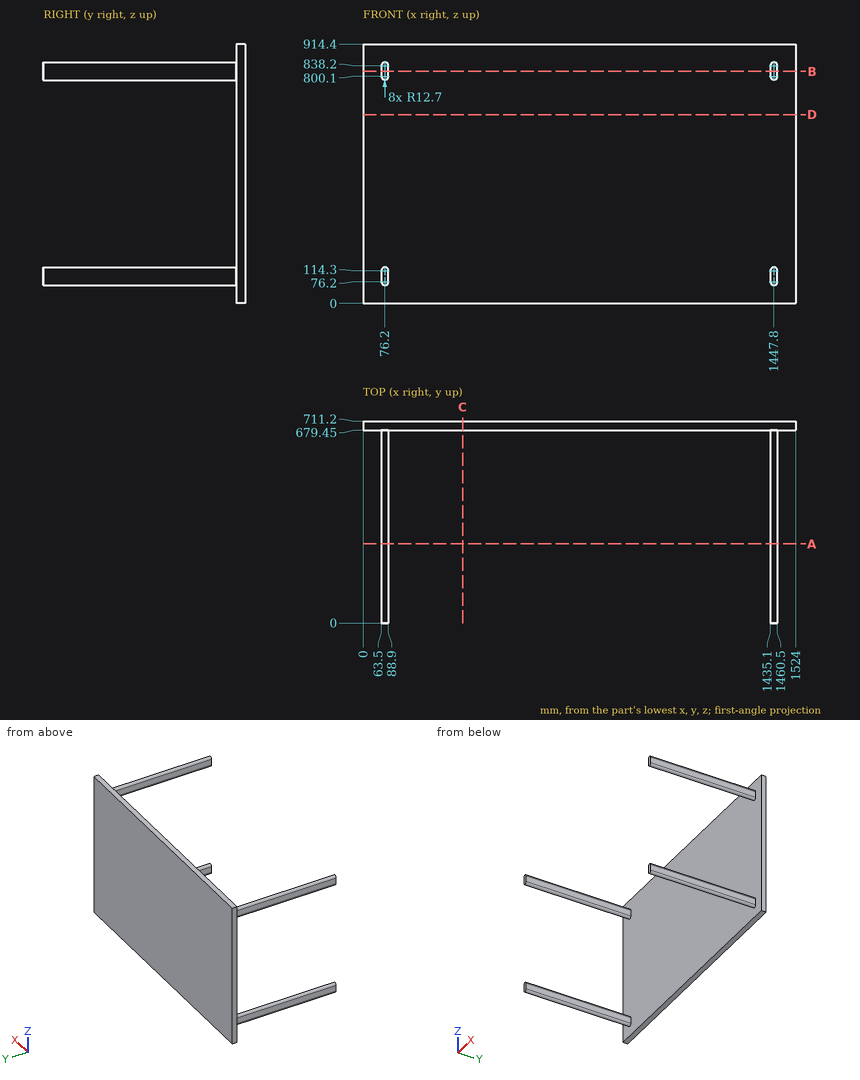
Print and shaded views of the part. All mm, measured from the part's lowest x, y and z. Give positions to 0.01 mm unless a question says otherwise; leave off trailing zeros. Write each loop counter-clockwise with the first axis right and the second up, starting at its lowest first coordinate (ties: lowest second). Pieces come first, ordered by that corner, then holes. Notation, with made-up numbers: (40.25, 60) - (45.25, 60) arc R18 ccw to (45.25, 92) - close; hole circle Ø2 at (-16, 44). An arc over 180 degrees is marked (long way). Put each result on its own line as item: value.
(1) Saw through at B-B (z = 817.5). List the corners of the cut face in (x, y), then the cut area to 3 significant figures.
Working result:
outline: (0, 679.45) - (63.5, 679.45) - (63.5, 0) - (88.9, 0) - (88.9, 679.45) - (1435.1, 679.45) - (1435.1, 0) - (1460.5, 0) - (1460.5, 679.45) - (1524, 679.45) - (1524, 711.2) - (0, 711.2) - close
area: 82,900 mm^2
(2) Drop flat-ended pins along their axis: pin 1 Ø4 at (x, z) = (445.5, 620.5) entering from -Y; pin 2 Ø11.5 at (y, z) = (273.5, 89) entering from -X; pin 3 Ø19 at (y, z) = (191.5, 88) entering from +X. Give the stop position or say it passes through.
Working result:
pin 1: y = 679.45
pin 2: x = 63.5
pin 3: x = 1460.5
(3) Wall check: L1, parallel to Y at x = 1180.5, z = 280.5; L2, parallel to X at y = 258.5, z = 94. Give the ranges that are in metal, low to high.
Working result:
L1: 679.45 to 711.2
L2: 63.5 to 88.9, 1435.1 to 1460.5
(4) Saw through at D-D (z = 665). List the corners of the cut face in (x, y).
Working result:
outline: (0, 679.45) - (1524, 679.45) - (1524, 711.2) - (0, 711.2) - close
(5) Saw through at A-A (y = 279.5). List the corners of the cut face in (x, z).
Working result:
outline: (63.5, 76.2) arc R12.7 ccw to (88.9, 76.2) - (88.9, 114.3) arc R12.7 ccw to (63.5, 114.3) - close; (63.5, 800.1) arc R12.7 ccw to (88.9, 800.1) - (88.9, 838.2) arc R12.7 ccw to (63.5, 838.2) - close; (1435.1, 76.2) arc R12.7 ccw to (1460.5, 76.2) - (1460.5, 114.3) arc R12.7 ccw to (1435.1, 114.3) - close; (1435.1, 800.1) arc R12.7 ccw to (1460.5, 800.1) - (1460.5, 838.2) arc R12.7 ccw to (1435.1, 838.2) - close
(6) Saw through at C-C (x = 350). List the corners of the cut face in (y, z).
Working result:
outline: (679.45, 0) - (711.2, 0) - (711.2, 914.4) - (679.45, 914.4) - close
